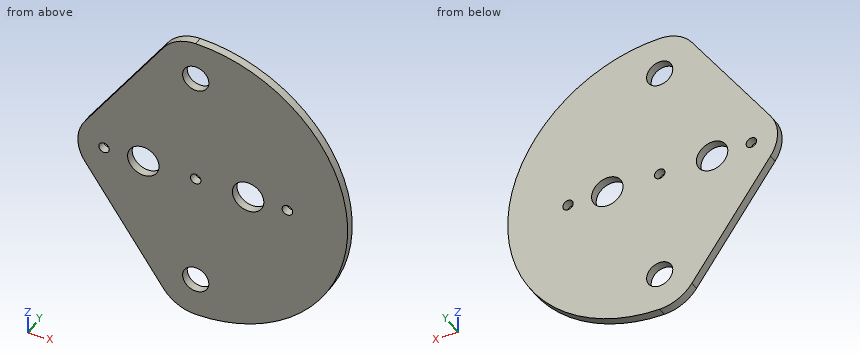
from build123d import *

# Parameters (mm, degrees)
SKETCH1_R           = 2.5
SKETCH1_R_2         = 3
SKETCH1_R_3         = 1
BOSS_EXTRUDE1_DEPTH = 0.8
BOSS_EXTRUDE2_DEPTH = 1.6


with BuildPart() as part:
    # Sketch1 → Boss-Extrude1 (new, symmetric)
    with BuildSketch(Plane(origin=(0, 0, 0), x_dir=(1, 0, 0), z_dir=(0, 1, 0))):
        with BuildLine():
            Line((-21.150952157, 4.29136197), (-6.150952157, 25.79136197))
            ThreePointArc((-6.150952157, 25.79136197), (0, 29), (6.150952157, 25.79136197))
            Line((6.150952157, 25.79136197), (21.150952157, 4.29136197))
            ThreePointArc((21.150952157, 4.29136197), (22.5, 0), (21.150952157, -4.29136197))
            Line((21.150952157, -4.29136197), (6.150952157, -25.79136197))
            ThreePointArc((6.150952157, -25.79136197), (0, -29), (-6.150952157, -25.79136197))
            Line((-6.150952157, -25.79136197), (-21.150952157, -4.29136197))
            ThreePointArc((-21.150952157, -4.29136197), (-22.5, 0), (-21.150952157, 4.29136197))
        make_face()
        with Locations(Location((0, 21.5, 0), (0, 0, 270))):
            Circle(SKETCH1_R, mode=Mode.SUBTRACT)
        with Locations(Location((0, -21.5, 0), (0, 0, 270))):
            Circle(SKETCH1_R, mode=Mode.SUBTRACT)
        with Locations(Location((-10, 0, 0), (0, 0, 270))):
            Circle(SKETCH1_R_2, mode=Mode.SUBTRACT)
        with Locations(Location((10, 0, 0), (0, 0, 270))):
            Circle(SKETCH1_R_2, mode=Mode.SUBTRACT)
        with Locations(Location((-17.5, 0, 0), (0, 0, 270))):
            Circle(SKETCH1_R_3, mode=Mode.SUBTRACT)
        with Locations(Location((0, 0, 0), (0, 0, 270))):
            Circle(SKETCH1_R_3, mode=Mode.SUBTRACT)
        with Locations(Location((17.5, 0, 0), (0, 0, 270))):
            Circle(SKETCH1_R_3, mode=Mode.SUBTRACT)
    extrude(amount=BOSS_EXTRUDE1_DEPTH, both=True)

    # Sketch2 → Boss-Extrude2 (add, through all)
    with BuildSketch(Plane(origin=(0, 0.8, 0), x_dir=(1, 0, 0), z_dir=(0, 1, 0))):
        with BuildLine():
            Line((0, -29), (22.5, 0))
            Line((22.5, 0), (0, 29))
            ThreePointArc((0, 29), (29, 0), (0, -29))
        make_face()
    extrude(amount=-BOSS_EXTRUDE2_DEPTH)


solid = part.part
Can you work these out from the model? Positions are in its coordinate system, mm. Round coordinates to 2 decimals unless told otherwise and drop trailing zeros. Order: outer loops, then holes, each group sorted by start corner. A loop starts at its lowest first (then second) coordinate and runs counter-clockwise, first axis right, second up. Notation, with made-up numbers: M 50,9 L 63,9 A36 cw 63,48 Z; hole C 67.5,64 d2. An arc over 180 degrees is marked long. Use a Markdown table: item, result.
1) Imagine slicing it at B-B (x = -17.5). List the corners of the cut face in (y, z) for me, then the cut area to 3 significant figures.
Geometry says:
| item | result |
|---|---|
| outline | M -0.8,-9.52 L 0.8,-9.52 L 0.8,-1 L -0.8,-1 Z; M -0.8,1 L 0.8,1 L 0.8,9.52 L -0.8,9.52 Z |
| area | 27.3 mm² |
2) Imagine slicing it at A-A (y = 0.15). List the corners of the cut face in (x, z) for me, then the cut area to 3 significant figures.
Geometry says:
| item | result |
|---|---|
| outline | M -21.15,-4.29 L -6.15,-25.79 A7.5 ccw 0,-29 A29 ccw 0,29 A7.5 ccw -6.15,25.79 L -21.15,4.29 A7.5 ccw Z; hole C -17.5,0 d2; hole C -10,0 d6; hole C 0,-21.5 d5; hole C 0,21.5 d5; hole C 0,0 d2; hole C 10,0 d6; hole C 17.5,0 d2 |
| area | 2,020 mm² |
3) Imagine slicing it at D-D (x = 14). List the corners of the cut face in (y, z) for me, then the cut area to 3 significant figures.
Geometry says:
| item | result |
|---|---|
| outline | M -0.8,-25.4 L 0.8,-25.4 L 0.8,25.4 L -0.8,25.4 Z |
| area | 81.3 mm² |
4) Imagine slicing it at C-C (z = -21.5). List the corners of the cut face in (x, y) for me, then the cut area to 3 significant figures.
Geometry says:
| item | result |
|---|---|
| outline | M -9.14,-0.8 L -2.5,-0.8 L -2.5,0.8 L -9.14,0.8 Z; M 2.5,-0.8 L 19.46,-0.8 L 19.46,0.8 L 2.5,0.8 Z |
| area | 37.8 mm² |
5) If I drill on line 1 along X through (y, z) = (-0.2, 0); line 2 along Z through (x, y) = (2, 0.75); line 3 along X through (y, z) = (0.05, 2.5), over which ranges is the centre line in solid material (lowest first)?
Geometry says:
| item | result |
|---|---|
| line 1 | x = -22.5 to -18.5, -16.5 to -13, -7 to -1, 1 to 7, 13 to 16.5, 18.5 to 29 |
| line 2 | z = -28.93 to -23, -20 to 20, 23 to 28.93 |
| line 3 | x = -22.07 to -11.66, -8.34 to 8.34, 11.66 to 28.89 |
